For this review, take the finished solid that the model builds, in its own axes (mm). A direction names the side the tool comes from. Round coordinates to 2 decimals unless told otherwise and drop trailing zeros. Loops run counter-clockwise (first coordinate to the right, second up) from the corner with the lowest first, then second, coordinate; pieces in that order, holes last. Notation, with made-up numbers: M 12.25,1 L 31.25,1 A18 ccw 31.25,12 Z; hole C 4,4 d11. An arc over 180 degrees is marked long. One line per question, with ' | ' between items. Start each with the question number.
1) Mouldability with a two-part tool opening along Z and no side actions: class faces 3 (the face through (-50, 346, 1)), 4 (the face through (1, 345, 50)), 5 (the face through (-1, 345, 47)), 6 (the face through (1, 345, -47)) as pulls with the +Z half, pulls with the -Z half, needs draft (parallel to the pull), parting line crosses it, or undercut.
2) We need section C-C (y = 451.5). Give the boundary of the cut face in (x, z), and give its area (3 significant figures).
3) For faces 1 (the face through (-47, 346, -1)), 2 (the face through (4, 46, -48)), list the 3-axis set-ups (+Z, -Z, +X, -X, +Y, -Y) from which the entire face can be reached by the end or side of a thin tool; tool diameter is ignored.
4) For probe 1 along X at (y, z) = (366.5, -3.5); probe 2 along Z at (x, y) = (45.5, 507), list the stretches that pass through material, from the lowest coordinate up. Write a range as from..to.
5) We need section B-B (x = 6). Give the boundary of the cut face in (y, z), and give its area (3 significant figures).
6) We need section D-D (y = 80). Give the boundary of the cut face in (x, z).
7) We need section A-A (z = -2). Give the boundary of the cut face in (x, y).
```python
from build123d import *

# Parameters (mm, degrees)
F1_DEPTH = 700
F4_DEPTH = 100.001
F5_DEPTH = 100.001


with BuildPart() as f1:
    # F0 (on Front) → F1 (new body)
    with BuildSketch(Plane.XZ):
        with BuildLine():
            ThreePointArc((50, 45), (48.5355339059, 48.5355339059), (45, 50))
            Line((45, 50), (-45, 50))
            ThreePointArc((-45, 50), (-48.5355339059, 48.5355339059), (-50, 45))
            Line((-50, 45), (-50, -45))
            ThreePointArc((-50, -45), (-48.5355339059, -48.5355339059), (-45, -50))
            Line((-45, -50), (45, -50))
            ThreePointArc((45, -50), (48.5355339059, -48.5355339059), (50, -45))
            Line((50, -45), (50, 45))
        make_face()
        with BuildLine():
            ThreePointArc((-47, 45), (-46.4142135624, 46.4142135624), (-45, 47))
            Line((-45, 47), (45, 47))
            ThreePointArc((45, 47), (46.4142135624, 46.4142135624), (47, 45))
            Line((47, 45), (47, -45))
            ThreePointArc((47, -45), (46.4142135624, -46.4142135624), (45, -47))
            Line((45, -47), (-45, -47))
            ThreePointArc((-45, -47), (-46.4142135624, -46.4142135624), (-47, -45))
            Line((-47, -45), (-47, 45))
        make_face(mode=Mode.SUBTRACT)
    extrude(amount=-F1_DEPTH)

    # F3 (on offset) → F4 (cut, through all)
    with BuildSketch(Plane.XY.offset(50)):
        Polygon((-50, 100), (-50, 0), (50, 0), align=None)
    extrude(amount=-F4_DEPTH, mode=Mode.SUBTRACT)

    # F3 (on offset) → F5 (cut, through all)
    with BuildSketch(Plane.XY.offset(50)):
        Polygon((-50, 100), (-50, 0), (50, 0), align=None)
        Polygon((50, 700), (-50, 700), (-50, 600), align=None)
    extrude(amount=-F5_DEPTH, mode=Mode.SUBTRACT)


solid = f1.part
```
Answers below:
1) face 3: needs draft | face 4: pulls with the +Z half | face 5: undercut | face 6: undercut
2) outline: M -50,-45 A5 ccw -45,-50 L 45,-50 A5 ccw 50,-45 L 50,45 A5 ccw 45,50 L -45,50 A5 ccw -50,45 Z; hole M -47,-45 A2 ccw -45,-47 L 45,-47 A2 ccw 47,-45 L 47,45 A2 ccw 45,47 L -45,47 A2 ccw -47,45 Z | area: 1,150 mm^2
3) face 1: +Y, -Y | face 2: +Z, -Z, -X, -Y
4) probe 1: -50..-47, 47..50 | probe 2: -49.97..-46.94, 46.94..49.97
5) outline: M 44,-50 L 656,-50 L 656,-47 L 44,-47 Z; M 44,47 L 656,47 L 656,50 L 44,50 Z | area: 3,670 mm^2
6) outline: M -30,-50 L 45,-50 A5 ccw 50,-45 L 50,45 A5 ccw 45,50 L -30,50 L -30,47 L 45,47 A2 cw 47,45 L 47,-45 A2 cw 45,-47 L -30,-47 Z
7) outline: M -50,100 L -47,97 L -47,603 L -50,600 Z; M 47,3 L 50,0 L 50,700 L 47,697 Z
